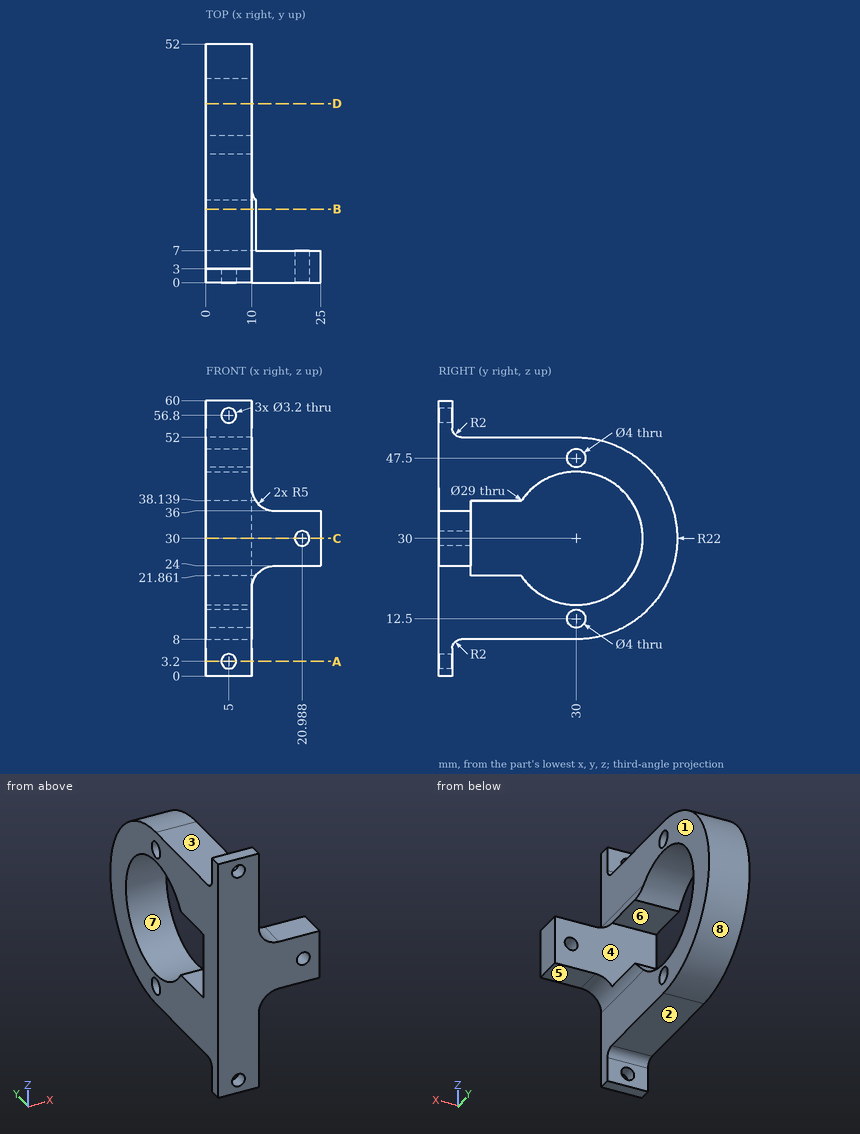
Input: dimensioned drawing with shaded views. Units: mm. Origin: part minimum x, y, z. A direction names the side the tool comes from. Coordinates: 2 decimals unless noted, no trailing zeros. Write each loop counter-clockwise with the first axis right and the second up, starting at its lowest first coordinate (ties: lowest second). Pieces come first, ordered by that corner, then holes. Notation, with made-up numbers: (5, 86) -> (60, 86) arc R17 cw to (60, 91) -> close; hole circle Ø5 at (11.5, -28.5). An arc over 180 degrees is marked (long way). Return JSON: item names as keys, results as strings. Group by question number.
1) Section query D-D, the plane y = 39. Return loops of the section in (x, z) (1 decimal), plus the area to 3 significant figures.
2) Section query C-C, the plane z = 30. Return loops of the section in (x, y), plus the area to 3 significant figures.
3) Set-up query: the marked faces 1, 2, 3 and 4. Return all of +Z, -Z, +X, -X, +Y, -Y with unobstructed straight access to the full face (end or side cutting, diameter ignored); none if empty.
4) Ray query, line 1 along X through (y, z) = (2, 30); line 2 along Y through (x, z) = (3.25, 30); line 3 along X through (y, z) = (2.45, 3.2). Return the intervals inside material, ascending.
5) Section query A-A, the plane z = 3.2. Return loops of the section in (x, y).
6) Mould query, pull axis Y, two halves, no side actions, for the marked faces 5, 6, 7 and 8. Classes: +Y half, -Y half, draft (parallel to the pull), parting line (faces both ways), or undercut.
7) Contact query for flat-ended pins moving along their axis: P1, Ø2, axis at x = 18.5, y = 4, coming from the -Z side; P2, Ø1.5, axis at x = 4.5, y = 15.5, coming from the -Z side; P3, Ø12, axis at x = 11, y = 41, coming from the -Z side (1 decimal). Output: stop coordinate, or through.
8) Section query B-B, the plane y = 16. Return loops of the section in (x, z).
From the geometry:
{
 "1": {"outline": "(0, 9.9) -> (10, 9.9) -> (10, 18.6) -> (0, 18.6) -> close; (0, 41.4) -> (10, 41.4) -> (10, 50.1) -> (0, 50.1) -> close", "area": "174 mm²"},
 "2": {"outline": "(0, 0) -> (19.39, 0) -> (19.39, 7) -> (0, 7) -> close; (0, 44.5) -> (10, 44.5) -> (10, 52) -> (0, 52) -> close; (22.59, 0) -> (25, 0) -> (25, 7) -> (22.59, 7) -> close", "area": "228 mm²"},
 "3": {"face 1": "+X, +Y", "face 2": "-Z, +X, -X, +Y", "face 3": "+Z, +X, -X, +Y", "face 4": "+X, -X"},
 "4": {"line 1": "0 to 19.39, 22.59 to 25", "line 2": "0 to 7, 44.5 to 52", "line 3": "0 to 3.4, 6.6 to 10"},
 "5": {"outline": "(0, 0) -> (3.4, 0) -> (3.4, 3) -> (0, 3) -> close; (6.6, 0) -> (10, 0) -> (10, 3) -> (6.6, 3) -> close"},
 "6": {"face 5": "draft", "face 6": "undercut", "face 7": "undercut", "face 8": "+Y half"},
 "7": {"P1": "z = 24", "P2": "z = 8", "P3": "z = 8.6"},
 "8": {"outline": "(0, 8) -> (10, 8) -> (10, 19) arc R5 cw to (10.9, 21.86) -> (0, 21.86) -> close; (0, 38.14) -> (10.9, 38.14) arc R5 cw to (10, 41) -> (10, 52) -> (0, 52) -> close"}
}
